Check sheet for the modelled part. Datum: model origin and axes. Units: mm. Round coordinates to 2 decimals unless told otherwise and drop trailing zeros. Order: outer loops, then holes, each group sorted by start corner. A loop starts at its lowest first (then second) coordinate and runs counter-clockwise, first axis right, second up.
(1) Sectioned sample at A-A, the plane z = -55. Enter the section's corners in (x, y), and give its area (3 significant figures).
(2) Depth check by flat-ended pin: pin 1 (2.5 mm diameter, centred on x = 178.5, y = 20.5, fed in from +Z); pin 2 (6.5 mm diameter, centred on x = 179, y = 21, fed in from +Z); pin 3 (1.2 mm diameter, centred on x = 177, y = 19, fed in from +Z). Enter the tip coordinate at first touch or a pass-through.
(3) Thickness scan on probe 1 along Z at (x, y) = (103.5, 26); probe 2 along Y at (x, z) = (119, -10); probe 3 along Y at (x, z) = (62.5, -70). Record the ranges inside material, lowest first.
```python
from build123d import *

# Parameters (mm, degrees)
SKETCH_1_W          = 150
SKETCH_1_H          = 90
EXTRUDE_1_DEPTH     = 35
SKETCH_2_R          = 5
EXTRUDE_2_DEPTH     = 1.8
FILLET_1_R          = 3
CHAMFER_1_SIZE      = 1
CHAMFER_2_SIZE      = 1.8
SKETCH_3_R          = 4.15
CUT_EXTRUDE_1_DEPTH = 5.8
SKETCH_4_R          = 0.75
EXTRUDE_3_DEPTH     = 5
CUT_EXTRUDE_2_DEPTH = 0.01
SKETCH_6_W          = 113
SKETCH_6_H          = 13
EXTRUDE_4_DEPTH     = 0.01


with BuildPart() as part:
    # 草图1 → 凸台-拉伸1 (new body)
    with BuildSketch(Plane(origin=(0, 0, 0), x_dir=(1, 0, 0), z_dir=(0, 1, 0))):
        with Locations((116.751230923, 45)):
            Rectangle(SKETCH_1_W, SKETCH_1_H)
    extrude(amount=EXTRUDE_1_DEPTH)

    # 草图2 → 凸台-拉伸2 (add)
    with BuildSketch(Plane.XZ):
        with Locations(Location((173.751230923, -18, 0), (0, 0, 90))):
            Circle(SKETCH_2_R)
        with Locations(Location((59.751230923, -18, 0), (0, 0, 90))):
            Circle(SKETCH_2_R)
        with Locations(Location((59.751230923, -72, 0), (0, 0, 90))):
            Circle(SKETCH_2_R)
        with Locations(Location((173.751230923, -72, 0), (0, 0, 90))):
            Circle(SKETCH_2_R)
    extrude(amount=EXTRUDE_2_DEPTH)

    # 圆角1
    fillet_1_edges = [part.edges().sort_by_distance(p)[0] for p in [
        (41.751230923, 17.5, -90),
        (191.751230923, 17.5, -90),
        (191.751230923, 17.5, 0),
        (41.751230923, 17.5, 0),
    ]]
    fillet(fillet_1_edges, radius=FILLET_1_R)

    # 倒角1
    chamfer_1_edges = [part.edges().sort_by_distance(p)[0] for p in [
        (191.751230923, 0, -45),
        (191.751230923, 35, -45),
        (41.751230923, 0, -45),
        (116.751230923, 0, -90),
        (116.751230923, 0, 0),
        (42.629910579, 0, -89.121320344),
        (42.629910579, 0, -0.878679656),
        (190.872551266, 0, -89.121320344),
        (190.872551266, 0, -0.878679656),
        (116.751230923, 35, 0),
        (41.751230923, 35, -45),
        (116.751230923, 35, -90),
        (42.629910579, 35, -89.121320344),
        (42.629910579, 35, -0.878679656),
        (190.872551266, 35, -89.121320344),
        (190.872551266, 35, -0.878679656),
    ]]
    chamfer(chamfer_1_edges, length=CHAMFER_1_SIZE)

    # 倒角2
    chamfer_2_edges = [part.edges().sort_by_distance(p)[0] for p in [
        (173.751230923, -1.8, -23),
        (59.751230923, -1.8, -23),
        (59.751230923, -1.8, -77),
        (173.751230923, -1.8, -77),
    ]]
    chamfer(chamfer_2_edges, length=CHAMFER_2_SIZE - 0.0001)  # a hair under: the kernel refuses the full size

    # 草图3 → 切除-拉伸1 (cut)
    with BuildSketch(Plane.XY):
        with Locations((176.751230923, 19)):
            Circle(SKETCH_3_R)
    extrude(amount=-CUT_EXTRUDE_1_DEPTH, mode=Mode.SUBTRACT)

    # 草图4 → 凸台-拉伸3 (add)
    with BuildSketch(Plane.XY.offset(-5.8)):
        with Locations((176.751230923, 19)):
            Circle(SKETCH_4_R)
    extrude(amount=EXTRUDE_3_DEPTH)

    # 草图5 → 切除-拉伸2 (cut)
    with BuildSketch(Plane.XY):
        Polygon((176.751230923, 23.5), (172.251230923, 23.5), (172.251230923, 12.5), (181.251230923, 12.5), (181.251230923, 23.5), align=None)
    extrude(amount=-CUT_EXTRUDE_2_DEPTH, mode=Mode.SUBTRACT)

    # 草图6 → 凸台-拉伸4 (add)
    with BuildSketch(Plane.XY):
        with Locations((113.251230923, 19)):
            Rectangle(SKETCH_6_W, SKETCH_6_H)
    extrude(amount=EXTRUDE_4_DEPTH)


solid = part.part
```
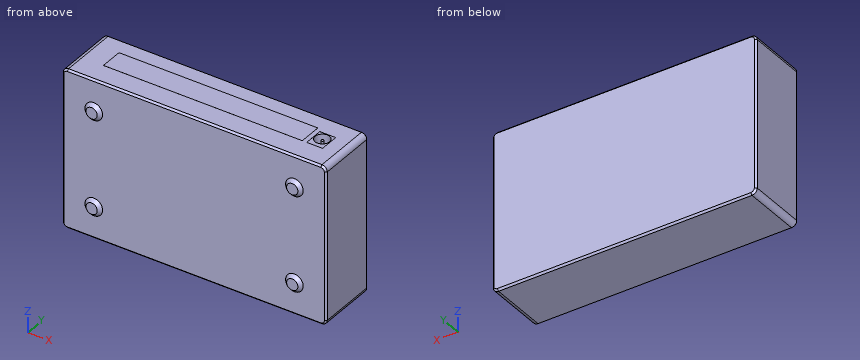
Derived:
1. outline: (41.75, 1) - (42.75, 0) - (190.75, 0) - (191.75, 1) - (191.75, 34) - (190.75, 35) - (42.75, 35) - (41.75, 34) - close
1. area: 5,250 mm2
2. pin 1: stops at z = -5.8
2. pin 2: stops at z = 0
2. pin 3: stops at z = -0.8
3. probe 1: z = -90 to 0
3. probe 2: y = 0 to 35
3. probe 3: y = -1.6 to 35
